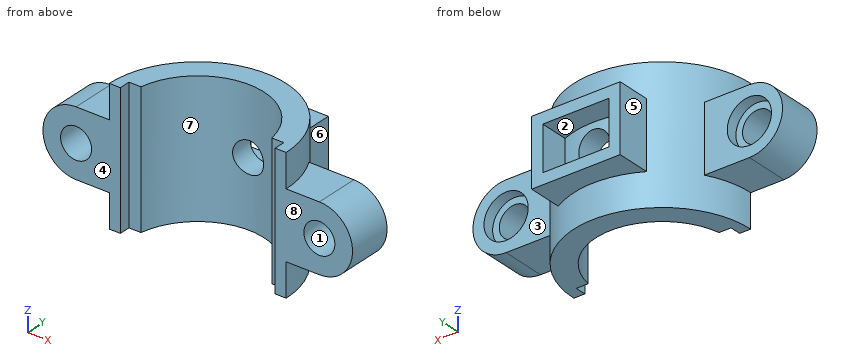
```python
from build123d import *

# Parameters (mm, degrees)
BOSS_EXTRUDE1_DEPTH      = 20
BOSS_EXTRUDE2_DEPTH      = 30
BOSS_EXTRUDE3_REACH      = 93.104
BOSS_EXTRUDE3_END_RADIUS = 40
SKETCH3_W                = 40
SKETCH3_H                = 30
SKETCH3_W_2              = 30
SKETCH3_H_2              = 20
CUT_EXTRUDE1_DEPTH       = 105.880884817
CUT_EXTRUDE1_DEPTH_BACK  = 105.880884817
SKETCH5_W                = 70
SKETCH5_H                = 5
CUT_EXTRUDE2_DEPTH       = 105.880884817
HOLE1_D                  = 14
HOLE3_D                  = 14
HOLE3_DEPTH              = 20
HOLE3_CBORE_D            = 20
HOLE3_CBORE_DEPTH        = 5
HOLE3_TIP                = 4.206024333


with BuildPart() as part:
    # Sketch1 → Boss-Extrude1 (new body)
    with BuildSketch(Plane(origin=(0, 0, 0), x_dir=(1, 0, 0), z_dir=(0, 1, 0))):
        with BuildLine():
            Line((-55, 15), (55, 15))
            ThreePointArc((55, 15), (70, 0), (55, -15))
            Line((55, -15), (-55, -15))
            ThreePointArc((-55, -15), (-70, 0), (-55, 15))
        make_face()
    extrude(amount=BOSS_EXTRUDE1_DEPTH)

    # Sketch2 → Boss-Extrude2 (add, symmetric)
    with BuildSketch(Plane.XY):
        with BuildLine():
            Line((-40, 0), (40, 0))
            ThreePointArc((40, 0), (0, 40), (-40, 0))
        make_face()
    extrude(amount=BOSS_EXTRUDE2_DEPTH, both=True)

    # Boss-Extrude3: up to this cylinder (the profile starts outside it)
    boss_extrude3_end = Plane(origin=(0, 0, -14.5), z_dir=(0, 0, -1)) * Cylinder(BOSS_EXTRUDE3_END_RADIUS, 267.208, mode=Mode.PRIVATE)
    # Sketch3 → Boss-Extrude3 (add, up to the surface)
    with BuildSketch(Plane(origin=(0, 50, 0), x_dir=(1, 0, 0), z_dir=(0, 1, 0)), mode=Mode.PRIVATE) as boss_extrude3_sk1:
        Rectangle(SKETCH3_W, SKETCH3_H)
        Rectangle(SKETCH3_W_2, SKETCH3_H_2, mode=Mode.SUBTRACT)
    boss_extrude3_tool1 = extrude(boss_extrude3_sk1.sketch, amount=-BOSS_EXTRUDE3_REACH, mode=Mode.PRIVATE) - boss_extrude3_end
    add(boss_extrude3_tool1.solids().sort_by_distance((0, 50, -14.5))[0])

    # Sketch4 → Cut-Extrude1 (cut, two sides: drawn at the far end of the back side and taken through both)
    with BuildSketch(Plane.XY.offset(30).offset(-CUT_EXTRUDE1_DEPTH_BACK)):
        with BuildLine():
            Line((-30, 0), (30, 0))
            ThreePointArc((30, 0), (0, 30), (-30, 0))
        make_face()
    extrude(amount=CUT_EXTRUDE1_DEPTH + CUT_EXTRUDE1_DEPTH_BACK, mode=Mode.SUBTRACT)

    # Sketch5 → Cut-Extrude2 (cut, through all)
    with BuildSketch(Plane.XY.offset(30)):
        with Locations((0, 2.5)):
            Rectangle(SKETCH5_W, SKETCH5_H)
    extrude(amount=-CUT_EXTRUDE2_DEPTH, mode=Mode.SUBTRACT)

    # Hole1 (through all)
    with Locations(Plane(origin=(0, 50, 0), x_dir=(1, 0, 0), z_dir=(0, 1, 0))):
        with Locations((0, 0)):
            Hole(HOLE1_D / 2)

    # Hole3
    with Locations(Plane(origin=(0, 20, 0), x_dir=(1, 0, 0), z_dir=(0, 1, 0))):
        with Locations((-55, 0), (55, 0)):
            CounterBoreHole(HOLE3_D / 2, HOLE3_CBORE_D / 2, HOLE3_CBORE_DEPTH, depth=HOLE3_DEPTH)
            with Locations((0, 0, -(HOLE3_DEPTH + HOLE3_TIP / 2))):  # 118° drill point
                Cone(0, HOLE3_D / 2, HOLE3_TIP, mode=Mode.SUBTRACT)


solid = part.part
```
CAD build for the part. Positions are in the model's coordinates, mm. Face numbers are marked on the shaded views. A direction names the side the tool comes from. Coordinates: 2 decimals unless noted, no trailing zeros. Write each loop counter-clockwise with the first axis right and the second up, starting at its lowest first coordinate (ties: lowest second). Pieces come first, ordered by that corner, then holes.
(1) Cut at C-C, the plane z = -18. List the corners of the cut face in (x, y).
(2) Cut at D-D, the plane x = -50.5. List the corners of the cut face in (y, z).
(3) Cut at A-A, the plane y = 17.5. List the corners of the cut face in (x, z), and give its area (3 significant figures).
(4) Flat gauge pins, fed straight in: pin 1 (10.5 mm diameter, centred on y = 46.5, z = 2.5, fed in from -X); pin 2 (6 mm diameter, centred on x = 51, z = -3.5, fed in from +Y); pin 3 (4 mm diameter, centred on y = 42, z = -5, fed in from +X); pin 4 (16 mm diameter, centred on x = -40.5, y = 9.5, fed in from +Z). Where does each tip first touch, or does it go through?
(5) Drill centre lines: probe 1 along Z at (x, y) = (14, 47); probe 2 along Z at (x, y) = (55, 9.75); probe 3 along X at (y, z) = (19, -3). Where is each one in solid material? Low to high.
(6) 3-axis set-ups, long thin cutter, end or side, ignore diameter. For the marked faces 1, 2, 3, 4 and 5: which of +Z, -Z, +X, -X, +Y, -Y reach the whole face in a straight line?
(7) Two-plate mould, pull along X, no slides. Class the marked faces 6, 7 and 8: +X half, -X half, draft (parallel to the pull), parting line (faces both ways), or undercut.
(8) Cut at B-B, the plane x = 0. List the corners of the cut face in (y, z), and give its area (3 significant figures).
Geometry says:
1. outline: (-40, 0) - (-35, 0) - (-35, 5) - (-29.58, 5) arc R30 cw to (29.58, 5) - (35, 5) - (35, 0) - (40, 0) arc R40 ccw to start
2. outline: (0, -15) - (20, -15) - (20, -8.93) - (15, -8.93) - (15, -5.36) - (0, -5.36) - close; (0, 5.36) - (15, 5.36) - (15, 8.93) - (20, 8.93) - (20, 15) - (0, 15) - close
3. outline: (-55, -15) - (-35.97, -15) - (-35.97, -30) - (-24.37, -30) - (-24.37, 30) - (-35.97, 30) - (-35.97, 15) - (-55, 15) arc R15 ccw to start; (24.37, -30) - (35.97, -30) - (35.97, -15) - (55, -15) arc R15 ccw to (55, 15) - (35.97, 15) - (35.97, 30) - (24.37, 30) - close; hole circle Ø20 at (-55, 0); hole circle Ø20 at (55, 0)
3. area: 2,610 mm2
4. pin 1: stops at x = -20
4. pin 2: stops at y = 15
4. pin 3: stops at x = 20
4. pin 4: stops at z = 30
5. probe 1: z = -15 to -10, 10 to 15
5. probe 2: z = -15 to -7, 7 to 15
5. probe 3: x = -69.7 to -64.54, -45.46 to -23.22, 23.22 to 45.46, 64.54 to 69.7
6. face 1: +Y, -Y
6. face 2: +Y
6. face 3: +Z, -Z, +X, +Y
6. face 4: +Z, -Z, +X, -X, -Y
6. face 5: +Z, -Z, -X, +Y
7. face 6: +X half
7. face 7: undercut
7. face 8: draft
8. outline: (30, -30) - (40, -30) - (40, -15) - (50, -15) - (50, -10) - (40, -10) - (40, -7) - (30, -7) - close; (30, 7) - (40, 7) - (40, 10) - (50, 10) - (50, 15) - (40, 15) - (40, 30) - (30, 30) - close
8. area: 560 mm2
